from build123d import *

# Parameters (mm, degrees)
F0_R     = 1.5875
F0_R_2   = 10.16
F1_DEPTH = 12.319
F2_T     = 2.54


# Not quite as in the source:
# - a shell that OpenCascade refuses in one call is made with other operations: the cavity is built on its own and cut out


with BuildPart() as f1:
    # F0 (on Front) → F1 (new body)
    with BuildSketch(Plane.XZ):
        with BuildLine():
            Line((9.9187, 16.2687), (-9.9187, 16.2687))
            ThreePointArc((-9.9187, 16.2687), (-14.4088280605, 14.4088280605), (-16.2687, 9.9187))
            Line((-16.2687, 9.9187), (-16.2687, -9.9187))
            ThreePointArc((-16.2687, -9.9187), (-14.4088280605, -14.4088280605), (-9.9187, -16.2687))
            Line((-9.9187, -16.2687), (9.9187, -16.2687))
            ThreePointArc((9.9187, -16.2687), (14.4088280605, -14.4088280605), (16.2687, -9.9187))
            Line((16.2687, -9.9187), (16.2687, 9.9187))
            ThreePointArc((16.2687, 9.9187), (14.4088280605, 14.4088280605), (9.9187, 16.2687))
        make_face()
        with Locations((-11.303, -11.303)):
            Circle(F0_R, mode=Mode.SUBTRACT)
        with Locations((11.303, -11.303)):
            Circle(F0_R, mode=Mode.SUBTRACT)
        Circle(F0_R_2, mode=Mode.SUBTRACT)
        with Locations((-11.303, 11.303)):
            Circle(F0_R, mode=Mode.SUBTRACT)
        with Locations((11.303, 11.303)):
            Circle(F0_R, mode=Mode.SUBTRACT)
    extrude(amount=F1_DEPTH)

    # F2: shell of thickness 2.54, made by hand


with BuildPart() as f2_core1:
    # F2_t2: copy of F1
    add(f1.part)

    # the walls: a layer under each face that stays
    f2_faces = [f2_core1.faces().sort_by_distance(p)[0] for p in [
        (14.4088280605, -6.1595, 14.4088280605),
        (-14.4088280605, -6.1595, 14.4088280605),
        (-14.4088280605, -6.1595, -14.4088280605),
        (14.4088280605, -6.1595, -14.4088280605),
        (-12.8905, -6.1595, -11.303),
        (9.7155, -6.1595, -11.303),
        (-10.16, -6.1595, 0),
        (-12.8905, -6.1595, 11.303),
        (9.7155, -6.1595, 11.303),
        (-10.8458, 0, 0),
        (-10.8458, -12.319, 0),
    ]]
    thicken(f2_faces, amount=-F2_T, mode=Mode.SUBTRACT)


with BuildPart() as f1_1:
    add(f1.part)

    # what is left inside the walls is the cavity
    f2_cavity = [f2_core1.part.solids().sort_by_distance(p)[0] for p in [
        (16.2433, -7.366, 0),
        (0, -7.366, 16.2433),
        (0, -7.366, -16.2433),
        (-16.2433, -7.366, 0),
    ]]
    add(f2_cavity, mode=Mode.SUBTRACT)


solid = f1_1.part
Geometry check sheet. Reference: the model listing, model coordinates, mm. A direction names the side the tool comes from. Round coordinates to 2 decimals unless told otherwise and drop trailing zeros. Loops run counter-clockwise (first coordinate to the right, second up) from the corner with the lowest first, then second, coordinate; pieces in that order, holes last. Notation, with made-up numbers: (77, 26.5) -> (106, 26.5) arc R18 ccw to (106, 53.5) -> close; hole circle Ø9 at (-2, -8.5). An arc over 180 degrees is marked (long way). Answer as a JSON object with one key per item and string values. Group by question number.
Item 1: Cross-section at A-A, the plane x = 0. Record the cut outline in (y, z), plus the area to 3 significant figures.
Item 2: Set-up check for faces 1 (the face through (16, -6, 9.919)), 2 (the face through (-14.359, -6.073, 14.458)): record each of +Z, -Z, +X, -X, +Y, -Y from which the full face is reachable in a straight line by a thin tool's end or side.
Item 3: Cross-section at D-D, the plane z = -14. Record the cut outline in (x, y), plus the area to 3 significant figures.
Item 4: Thickness scan on line 1 along Y through (x, z) = (1, 14.5); line 2 along Z through (x, y) = (12.5, -2.5); line 3 along Z through (x, y) = (11, -3.75). Record the ranges inside material, lowest first.
Item 5: Cross-section at B-B, the plane z = 0. Record the cut outline in (x, y), plus the area to 3 significant figures.
Item 6: Release check for a two-part mould opening along Z. For faces 3 (the face through (0, -1, -16.269)), 4 (the face through (16.269, -11, 0)), 5 (the face through (-16, -6, -9.919)), 6 (the face through (13.338, -6.109, -7.712)) record: pulls with the +Z half, pulls with the -Z half, needs draft (parallel to the pull), parting line crosses it, or undercut.
Item 7: Cross-section at C-C, the plane y = -10.5. Count the separate pieces of the cut face and the enclosed holes in it, plus the area to 3 significant figures.
Item 8: Depth check by flat-ended pin: pin 1 Ø1.2 at (y, z) = (-6.5, -16) entering from -X; pin 2 Ø1.5 at (y, z) = (-6.5, 1) entering from -X; pin 3 Ø0.5 at (y, z) = (-7.5, -16) entering from +X. Enter the tip coordinate at first touch or a pass-through.
Determined:
{
 "1": {"outline": "(-12.32, -16.27) -> (-9.78, -16.27) -> (-9.78, -12.7) -> (-2.54, -12.7) -> (-2.54, -16.27) -> (0, -16.27) -> (0, -10.16) -> (-12.32, -10.16) -> close; (-12.32, 10.16) -> (0, 10.16) -> (0, 16.27) -> (-2.54, 16.27) -> (-2.54, 12.7) -> (-9.78, 12.7) -> (-9.78, 16.27) -> (-12.32, 16.27) -> close", "area": "98.8 mm²"},
 "2": {"face 1": "+X", "face 2": "+Z, -X, +Y, -Y"},
 "3": {"outline": "(-14.78, -12.32) -> (14.78, -12.32) -> (14.78, 0) -> (-14.78, 0) -> close; hole (-8.18, -9.78) -> (8.18, -9.78) -> (8.18, -2.54) -> (-8.18, -2.54) -> close", "area": "246 mm²"},
 "4": {"line 1": "y = -12.32 to -9.78, -2.54 to 0", "line 2": "z = -15.72 to -12.35, -10.26 to 10.26, 12.35 to 15.72", "line 3": "z = -16.18 to -12.86, -9.74 to -7.19, -6.35 to 6.35, 7.19 to 9.74, 12.86 to 16.18"},
 "5": {"outline": "(-16.27, -12.32) -> (-10.16, -12.32) -> (-10.16, 0) -> (-16.27, 0) -> (-16.27, -2.54) -> (-12.7, -2.54) -> (-12.7, -9.78) -> (-16.27, -9.78) -> close; (10.16, -12.32) -> (16.27, -12.32) -> (16.27, -9.78) -> (12.7, -9.78) -> (12.7, -2.54) -> (16.27, -2.54) -> (16.27, 0) -> (10.16, 0) -> close", "area": "98.8 mm²"},
 "6": {"face 3": "pulls with the -Z half", "face 4": "needs draft", "face 5": "undercut", "face 6": "undercut"},
 "7": {"separate pieces": "1", "enclosed holes": "5", "area": "668 mm²"},
 "8": {"pin 1": "stops at x = -13.12", "pin 2": "stops at x = -12.7", "pin 3": "stops at x = 12.43"}
}
